Check sheet for the modelled part. Datum: model origin and axes. Units: mm. A direction names the side the tool comes from. Give positions to 0.01 mm unless a question says otherwise; leave off trailing zeros. Loops run counter-clockwise (first coordinate to the right, second up) from the corner with the lowest first, then second, coordinate; pieces in that order, holes last.
```python
from build123d import *

# Parameters (mm, degrees)
SKETCH1_W                      = 42
SKETCH1_H                      = 100
BOSS_EXTRUDE1_DEPTH            = 10
CUT_EXTRUDE1_DEPTH             = 56.145262716
F_2_5_2_5_DIAMETER_HOLE1_D     = 2.5
F_2_5_2_5_DIAMETER_HOLE2_D     = 2.5
F_2_5_2_5_DIAMETER_HOLE2_DEPTH = 7.5
F_2_5_2_5_DIAMETER_HOLE2_TIP   = 0.751075774


# Read off the part's stored shape, not the designer's step: CBORE for M6 Hex Head Bolt1
with BuildPart() as part:
    # Sketch1 → Boss-Extrude1 (new body)
    with BuildSketch(Plane.XY.offset(10)):
        Rectangle(SKETCH1_W, SKETCH1_H)
    extrude(amount=-BOSS_EXTRUDE1_DEPTH)

    # Sketch2 → Cut-Extrude1 (cut, through all)
    with BuildSketch(Plane(origin=(0, 0, 0), x_dir=(-1, 0, 0), z_dir=(0, 0, -1))):
        with BuildLine():
            Line((5.04, -6), (-6, -6))
            ThreePointArc((-6, -6), (-12, -12), (-6, -18))
            Line((-6, -18), (5.04, -18))
            ThreePointArc((5.04, -18), (11.04, -12), (5.04, -6))
        make_face()
    extrude(amount=-CUT_EXTRUDE1_DEPTH, mode=Mode.SUBTRACT)

    # Ø2.5 (2.5) Diameter Hole1 (through all)
    with Locations(Plane.XY.offset(10)):
        with Locations((13, 42), (-11, 42), (-11, -42), (13, -42)):
            Hole(F_2_5_2_5_DIAMETER_HOLE1_D / 2)

    # CBORE for M6 Hex Head Bolt1 outline → CBORE for M6 Hex Head Bolt1 (revolve, cut)
    with BuildSketch(Plane(origin=(0, -12, 5), x_dir=(0, 1, 0), z_dir=(0, 0, -1))):
        Polygon((3.5, -16), (3.5, -9.913035616), (0, -9.913035616), (0, -21), (4.5, -21), (4.5, -16), align=None)
    revolve(axis=Axis((0, -12, 5), (1, 0, 0)), mode=Mode.SUBTRACT)

    # Ø2.5 (2.5) Diameter Hole2
    with Locations(Plane.ZY.offset(21)):
        with Locations((5, 45), (5, -45)):
            Hole(F_2_5_2_5_DIAMETER_HOLE2_D / 2, depth=F_2_5_2_5_DIAMETER_HOLE2_DEPTH)
            with Locations((0, 0, -(F_2_5_2_5_DIAMETER_HOLE2_DEPTH + F_2_5_2_5_DIAMETER_HOLE2_TIP / 2))):  # 118° drill point
                Cone(0, F_2_5_2_5_DIAMETER_HOLE2_D / 2, F_2_5_2_5_DIAMETER_HOLE2_TIP, mode=Mode.SUBTRACT)


solid = part.part
```
(1) Section check D-D on y = 42. Record the boundary of the cut face in (x, z).
(2) Material ranges on line 1 (Y direction, x = 13, z = 5.5); line 2 (Y direction, x = -15.5, z = 5); line 3 (Y direction, x = -2.5, z = 1.5), recorded low to high.
(3) Access from +Z, -Z, +X, -X, +Y, -Y to the whole of each face (thin tool, end or side, straight path). Record for faces 5 (the face through (-12.914, -8.767, 3.659)), 6 (the face through (-9.72, -8.245, 4.93)), 7 (the face through (0, 1, 0)).
(4) Section check C-C on x = -17.5. Record the boundary of the cut face in (y, z).
(5) Release check for a two-part mould opening along Y. For faces 1 (the face through (0, -6, 5)), 2 (the face through (-21, -1, 5)), 3 (the face through (0, -50, 5)), 4 (the face through (0, 50, 5)) record: pulls with the +Y half, pulls with the -Y half, needs draft (parallel to the pull), parting line crosses it, or undercut.
(6) Section check A-A on x = -1.5. Record the boundary of the cut face in (y, z), plus the area to 3 significant figures.
(7) Section check B-B on y = -12. Record the boundary of the cut face in (x, z), plus the area to 3 significant figures.
(8) Gauge pin test, flat end, axial feed: pin 1 Ø2 at (y, z) = (45, 5) entering from -X. Record the tip position at first contact, or that the pin passes through.
Computed values:
1. outline: (-21, 0) - (-12.25, 0) - (-12.25, 10) - (-21, 10) - close; (-9.75, 0) - (11.75, 0) - (11.75, 10) - (-9.75, 10) - close; (14.25, 0) - (21, 0) - (21, 10) - (14.25, 10) - close
2. line 1: y = -50 to -43.25, -40.75 to 40.75, 43.25 to 50
2. line 2: y = -50 to -46.25, -43.75 to -15.5, -8.5 to 43.75, 46.25 to 50
2. line 3: y = -50 to -18, -6 to 50
3. face 5: -X
3. face 6: +Z, -Z
3. face 7: -Z, +X, -X, +Y, -Y
4. outline: (-50, 0) - (50, 0) - (50, 10) - (-50, 10) - close; hole circle Ø2.5 at (-45, 5); hole circle Ø9 at (-12, 5); hole circle Ø2.5 at (45, 5)
5. face 1: undercut
5. face 2: needs draft
5. face 3: pulls with the -Y half
5. face 4: pulls with the +Y half
6. outline: (-50, 0) - (-18, 0) - (-18, 10) - (-50, 10) - close; (-6, 0) - (50, 0) - (50, 10) - (-6, 10) - close
6. area: 880 mm2
7. outline: (-21, 0) - (-11.04, 0) - (-11.04, 1.5) - (-16, 1.5) - (-16, 0.5) - (-21, 0.5) - close; (-21, 9.5) - (-16, 9.5) - (-16, 8.5) - (-11.04, 8.5) - (-11.04, 10) - (-21, 10) - close; (12, 0) - (21, 0) - (21, 10) - (12, 10) - close
7. area: 110 mm2
8. pin 1: stops at x = -13.35
